Check sheet for the modelled part. Datum: model origin and axes. Units: mm. Face numbers are marked on the shaded views. Give positions to 0.01 mm unless a question says otherwise; leave off trailing zeros. Order: outer loops, then holes, each group sorted by start corner. A loop starts at its lowest first (then second) coordinate and runs counter-clockwise, first axis right, second up.
from build123d import *

# Parameters (mm, degrees)
F0_R     = 5.1
F0_R_2   = 1.1
F1_DEPTH = 20
F2_R     = 2
F3_SIZE  = 0.6


with BuildPart() as f1:
    # F0 (on Top) → F1 (new body)
    with BuildSketch(Plane.XY):
        Circle(F0_R)
        Circle(F0_R_2, mode=Mode.SUBTRACT)
    extrude(amount=F1_DEPTH)

    # F2
    f2_edges = [f1.edges().sort_by_distance(p)[0] for p in [
        (-5.1, 0, 20),
        (-5.1, 0, 0),
    ]]
    fillet(f2_edges, radius=F2_R)

    # F3
    f3_edges = [f1.edges().sort_by_distance(p)[0] for p in [
        (-1.1, 0, 20),
        (-1.1, 0, 0),
    ]]
    chamfer(f3_edges, length=F3_SIZE)


solid = f1.part
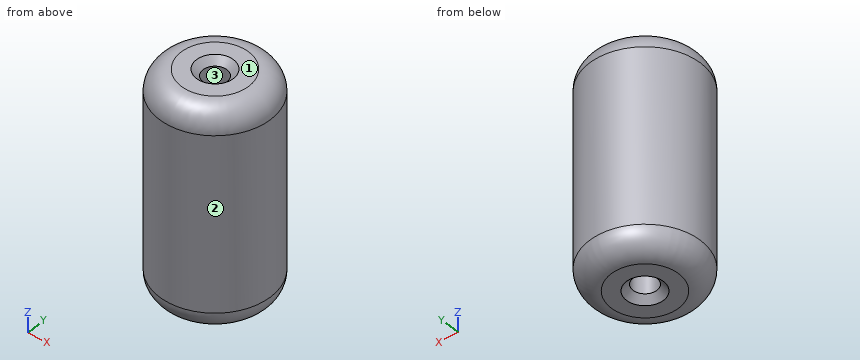
1) Draft check along X on the marked faces 1, 2 and 3. Enter one of: +X half, -X half, draft (parallel to the pull), parting line (faces both ways), or undercut.
Recorded:
face 1: draft
face 2: parting line
face 3: undercut
2) Depth check by flat-ended pin: pin 1 Ø2 at (x, y) = (-1, 0.5) entering from -Z; pin 2 Ø1.8 at (x, y) = (0, 0) entering from -Z; pin 3 Ø1 at (x, z) = (3, 8.5) entering from +Y. Enter the tip coordinate at first touch or a pass-through.
Recorded:
pin 1: stops at z = 0
pin 2: passes through
pin 3: stops at y = 4.45
3) Section check A-A, the plane y = 0. Record the cut outline in (x, z).
Recorded:
outline: (-5.1, 2) arc R2 ccw to (-3.1, 0) - (-1.7, 0) - (-1.1, 0.6) - (-1.1, 19.4) - (-1.7, 20) - (-3.1, 20) arc R2 ccw to (-5.1, 18) - close; (1.1, 0.6) - (1.7, 0) - (3.1, 0) arc R2 ccw to (5.1, 2) - (5.1, 18) arc R2 ccw to (3.1, 20) - (1.7, 20) - (1.1, 19.4) - close
4) Section check C-C, the plane z = 9. Record the cut outline in (x, y).
Recorded:
outline: circle Ø10.2 at (0, 0); hole circle Ø2.2 at (0, 0)
5) Material ranges on L1, parallel to Y at x = 0, z = 4.5; L2, parallel to X at y = -1, z = 9.5; L3, parallel to X at y = -0.5, z = 11.25, recorded low to high.
Recorded:
L1: y = -5.1 to -1.1, 1.1 to 5.1
L2: x = -5 to -0.46, 0.46 to 5
L3: x = -5.08 to -0.98, 0.98 to 5.08
